The model under review builds one solid part; all positions refer to its coordinate system, in mm. Coordinates: 2 decimals unless noted, no trailing zeros. Write each loop counter-clockwise with the first axis right and the second up, starting at its lowest first coordinate (ties: lowest second). Pieces come first, ordered by that corner, then holes. Notation, with made-up numbers: M -23,74 L -13,74 A17 cw -13,96 Z; hole C 72.25,59 d2. An arc over 180 degrees is marked long. Answer as a JSON object with one key per item and string values.
```python
from build123d import *

# Parameters (mm, degrees)
SKETCH_1_W                      = 200
SKETCH_1_H                      = 20
EXTRUDE_1_DEPTH                 = 30
SKETCH_3_W                      = 30
SKETCH_3_H                      = 17.724954358
EXTRUDE_2_DEPTH                 = 30
EXTRUDE_2_DEPTH_BACK            = 1
CUT_EXTRUDE_1_DEPTH             = 18
HOLE_WIZARD_G1_16_1_D           = 6.6
HOLE_WIZARD_G1_16_1_DEPTH       = 17.724954357
HOLE_WIZARD_G1_16_1_CSINK_D     = 7.773
HOLE_WIZARD_G1_16_1_CSINK_ANGLE = 90
SKETCH_9_W                      = 30
SKETCH_9_H                      = 17.724954358
EXTRUDE_3_DEPTH                 = 30
CUT_EXTRUDE_2_DEPTH             = 30
HOLE_WIZARD_G1_16_2_D           = 6.6
HOLE_WIZARD_G1_16_2_DEPTH       = 17.724954357
HOLE_WIZARD_G1_16_2_CSINK_D     = 7.773
HOLE_WIZARD_G1_16_2_CSINK_ANGLE = 90
SKETCH_14_W                     = 30
SKETCH_14_H                     = 1.0813423
SKETCH_14_H_2                   = 1.193703342
CUT_EXTRUDE_3_DEPTH             = 215


with BuildPart() as part:
    # 草图1 → 凸台-拉伸1 (new body)
    with BuildSketch(Plane(origin=(0, 0, 0), x_dir=(0, 0, -1), z_dir=(1, 0, 0))):
        with Locations((100, -10)):
            Rectangle(SKETCH_1_W, SKETCH_1_H)
    extrude(amount=EXTRUDE_1_DEPTH)

    # 草图3 → 凸台-拉伸2 (add, two sides)
    with BuildSketch(Plane.XY) as extrude_2_sk:
        with Locations((15, -9.943819479)):
            Rectangle(SKETCH_3_W, SKETCH_3_H)
    extrude(amount=EXTRUDE_2_DEPTH)
    extrude(extrude_2_sk.sketch, amount=-EXTRUDE_2_DEPTH_BACK)

    # 草图5 → 切除-拉伸1 (cut)
    with BuildSketch(Plane(origin=(0, -1.0813423, 0), x_dir=(1, 0, 0), z_dir=(0, 1, 0))):
        with BuildLine():
            ThreePointArc((15, -30), (4.393398282, -25.606601718), (0, -15))
            Line((0, -15), (0, -30))
            Line((0, -30), (15, -30))
        make_face()
        with BuildLine():
            Line((30, -30), (30, -15))
            ThreePointArc((30, -15), (25.606601718, -25.606601718), (15, -30))
            Line((15, -30), (30, -30))
        make_face()
    extrude(amount=-CUT_EXTRUDE_1_DEPTH, mode=Mode.SUBTRACT)

    # G1/16 螺纹孔1
    with Locations(Plane(origin=(0, -1.0813423, 0), x_dir=(1, 0, 0), z_dir=(0, 1, 0))):
        with Locations((15, -20.203891656)):
            CounterSinkHole(HOLE_WIZARD_G1_16_1_D / 2, HOLE_WIZARD_G1_16_1_CSINK_D / 2, depth=HOLE_WIZARD_G1_16_1_DEPTH, counter_sink_angle=HOLE_WIZARD_G1_16_1_CSINK_ANGLE)

    # 草图9 → 凸台-拉伸3 (add)
    with BuildSketch(Plane(origin=(0, 0, -200), x_dir=(-1, 0, 0), z_dir=(0, 0, -1))):
        with Locations((-15, -9.943819479)):
            Rectangle(SKETCH_9_W, SKETCH_9_H)
    extrude(amount=EXTRUDE_3_DEPTH)

    # 草图10 → 切除-拉伸2 (cut)
    with BuildSketch(Plane(origin=(0, -1.0813423, 0), x_dir=(1, 0, 0), z_dir=(0, 1, 0))):
        with BuildLine():
            Line((0, 230), (0, 215.122561862))
            ThreePointArc((0, 215.122561862), (3.737143337, 225.029532125), (13.086407972, 230))
            Line((13.086407972, 230), (0, 230))
        make_face()
        with BuildLine():
            ThreePointArc((16.913592028, 230), (26.262856663, 225.029532125), (30, 215.122561862))
            Line((30, 215.122561862), (30, 230))
            Line((30, 230), (16.913592028, 230))
        make_face()
    extrude(amount=-CUT_EXTRUDE_2_DEPTH, mode=Mode.SUBTRACT)

    # G1/16 螺纹孔2
    with Locations(Plane(origin=(0, -1.0813423, 0), x_dir=(1, 0, 0), z_dir=(0, 1, 0))):
        with Locations((15, 219.701584922)):
            CounterSinkHole(HOLE_WIZARD_G1_16_2_D / 2, HOLE_WIZARD_G1_16_2_CSINK_D / 2, depth=HOLE_WIZARD_G1_16_2_DEPTH, counter_sink_angle=HOLE_WIZARD_G1_16_2_CSINK_ANGLE)

    # 草图14 → 切除-拉伸3 (cut)
    with BuildSketch(Plane.XY):
        with Locations((15, -0.54067115)):
            Rectangle(SKETCH_14_W, SKETCH_14_H)
        with Locations((15, -19.403148329)):
            Rectangle(SKETCH_14_W, SKETCH_14_H_2)
    extrude(amount=-CUT_EXTRUDE_3_DEPTH, mode=Mode.SUBTRACT)


solid = part.part
```
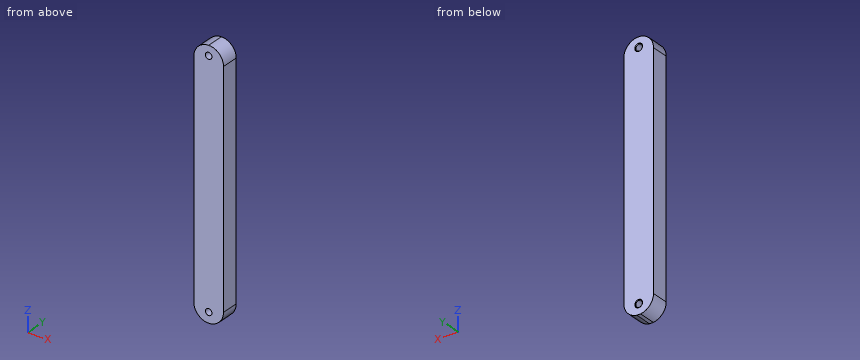
(1) Add section B-B on x = 24.5. Give the boundary of the cut face in (y, z).
Results list:
{"outline": "M -18.81,-226.73 L -1.08,-226.73 L -1.08,26.61 L -18.81,26.61 Z"}
(2) For pin 1 Ø6 at (x, y) = (10.5, -14) entering from +Z; pin 2 Ø2 at (x, y) = (11, -16) entering from -Z; pin 3 Ø3 at (x, y) = (25.5, -11.5) entering from +Z, all flat-tipped, find the tip position at first contact; note any pin that passes through.
Results list:
{"pin 1": "z = 29.92", "pin 2": "z = -229.82", "pin 3": "z = 27"}
(3) Add section A-A on y = -6.75. Give the boundary of the cut face in (x, z), and give its area (3 significant figures).
Results list:
{"outline": "M 0,-215.12 A15 ccw 13.09,-230 L 16.91,-230 A15 ccw 30,-215.12 L 30,15 A15 ccw 0,15 Z; hole C 15,-219.7 d6.6; hole C 15,20.2 d6.6", "area": "7,540 mm²"}
(4) Add section C-C on x = 4.5. Give the boundary of the cut face in (y, z).
Results list:
{"outline": "M -18.81,-225.83 L -1.08,-225.83 L -1.08,25.71 L -18.81,25.71 Z"}
(5) Wall thickness on line 1 along Z through (x, y) = (15, -11); line 2 along Z through (x, y) = (20.5, -17.5); line 3 along Z through (x, y) = (3.5, -9): over which ranges is each line inside the solid? List them lowest first. Write a range as from..to.
Results list:
{"line 1": "-230..-223, -216.4..16.9, 23.5..30", "line 2": "-229.08..28.96", "line 3": "-224.75..24.63"}
